Build history of the part. All positions in model axes, mm. Face numbers are marked on the shaded views. A direction names the side the tool comes from. Round coordinates to 2 decimals unless told otherwise and drop trailing zeros. Order: outer loops, then holes, each group sorted by start corner. A loop starts at its lowest first (then second) coordinate and runs counter-clockwise, first axis right, second up. Notation, with made-up numbers: (-11, 61.5) -> (-3, 61.5) arc R20 ccw to (-3, 88.5) -> close; hole circle Ø7 at (-16.75, -19). An arc over 180 degrees is marked (long way). Answer as a JSON object with one key per item and string values.
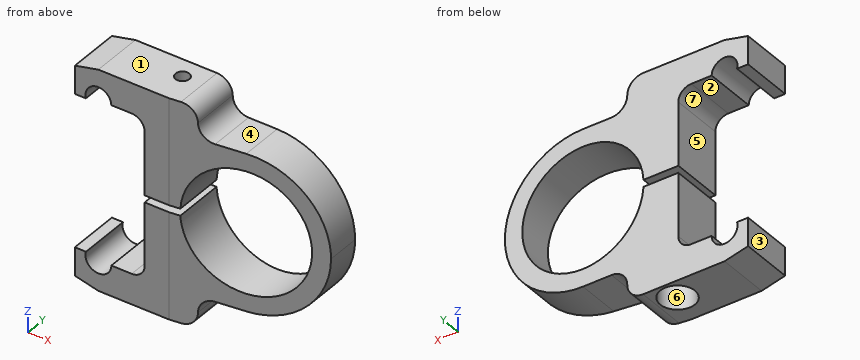
from build123d import *

# Parameters (mm, degrees)
F1_DEPTH       = 9.525
F3_D           = 2.54
F3_CBORE_D     = 6.35
F3_CBORE_DEPTH = 4.7752
F5_DEPTH       = 20.32


with BuildPart() as f1:
    # F0 (on Front) → F1 (new body)
    with BuildSketch(Plane.XZ):
        with BuildLine():
            ThreePointArc((-28.2059340648, 13.9065), (-26.240179578, 16.8438540599), (-23.5585, 14.5415))
            Line((-23.5585, 14.5415), (-19.8247, 14.5415))
            ThreePointArc((-19.8247, 14.5415), (-18.1543723615, 13.8496276385), (-17.4625, 12.1793))
            Line((-17.4625, 12.1793), (-17.4625, 0.6350352715))
            Line((-17.4625, 0.6350352715), (-11.0877819096, 0.6350352715))
            ThreePointArc((-11.0877819096, 0.6350352715), (11.0996948974, 3.52715e-05), (-11.0877819096, -0.6349647285))
            Line((-11.0877819096, -0.6349647285), (-17.4559396015, -0.6349647285))
            Line((-17.4559396015, -0.6349647285), (-17.4559396015, -12.1792647285))
            ThreePointArc((-17.4559396015, -12.1792647285), (-18.147811963, -13.8495923671), (-19.8181396015, -14.5414647285))
            Line((-19.8181396015, -14.5414647285), (-23.5519396015, -14.5414647285))
            ThreePointArc((-23.5519396015, -14.5414647285), (-26.2413382061, -16.9011545192), (-28.1991546105, -13.9065))
            Line((-28.1991546105, -13.9065), (-30.2311546105, -13.9065))
            Line((-30.2311546105, -13.9065), (-30.2311546105, -19.0742111302))
            Line((-30.2311546105, -19.0742111302), (-25.92066586, -20.0914))
            Line((-25.92066586, -20.0914), (-11.0116051104, -20.0914))
            ThreePointArc((-11.0116051104, -20.0914), (-8.9619217104, -19.2410649878), (-8.116123004, -17.1895055269))
            ThreePointArc((-8.116123004, -17.1895055269), (-7.2702919293, -15.137867554), (-5.220530089, -14.2875))
            Line((-5.220530089, -14.2875), (0, -14.2875))
            ThreePointArc((0, -14.2875), (10.1027881362, -10.1027881362), (14.2875, 0))
            ThreePointArc((14.2875, 0), (10.1027881362, 10.1027881362), (0, 14.2875))
            Line((0, 14.2875), (-5.220530089, 14.2875))
            ThreePointArc((-5.220530089, 14.2875), (-7.2612916673, 15.1288868805), (-8.1160675997, 17.1640767507))
            ThreePointArc((-8.1160675997, 17.1640767507), (-8.9646092373, 19.1930542961), (-10.9940030066, 20.0406))
            Line((-10.9940030066, 20.0406), (-25.92066586, 20.0406))
            Line((-25.92066586, 20.0406), (-30.2311546105, 19.0322602705))
            Line((-30.2311546105, 19.0322602705), (-30.2311546105, 13.9065))
            Line((-30.2311546105, 13.9065), (-28.2059340648, 13.9065))
        make_face()
    extrude(amount=F1_DEPTH)

    # F3 (through all)
    with Locations(Plane(origin=(0, 0, -20.0914), x_dir=(1, 0, 0), z_dir=(0, 0, -1))):
        with Locations((-14.6946051104, 3.683)):
            CounterBoreHole(F3_D / 2, F3_CBORE_D / 2, F3_CBORE_DEPTH)

    # F4 (on Top) → F5 (cut, symmetric)
    with BuildSketch(Plane.XY):
        Polygon((14.5003534853, -6.1715153816), (-13.6252772063, -9.5990113914), (14.5003534853, -10.0196320564), align=None)
    extrude(amount=F5_DEPTH, both=True, mode=Mode.SUBTRACT)


solid = f1.part
1) Cut at D-D, the plane z = -10.5. Give the cut face in (x, y) (3 decimals), plus the area to 3 significant figures.
Checked values:
{"outline": "(-17.456, -9.525) -> (-13.018, -9.525) -> (-3.612, -8.379) -> (-3.612, 0) -> (-17.456, 0) -> close; (3.605, -7.499) -> (9.689, -6.758) -> (9.689, 0) -> (3.605, 0) -> close; hole circle Ø2.54 at (-14.695, -3.683)", "area": "165 mm²"}
2) Probe L1, parallel to X at y = -3.25, z = -1.5; L2, parallel to X at y = -3.75, z = 6.5; L3, parallel to Z at x = -21.5, y = -3. List the from-to ranges inside material, lowest first. Write a range as from..to.
Checked values:
{"L1": "x = -17.46..-15.89, -13.5..-11, 11..14.21", "L2": "x = -17.46..-15.96, -13.43..-9, 9..12.72", "L3": "z = -20.09..-14.54, 14.54..20.04"}
3) Cut at C-C, the plane z = 13. Give the cut face in (x, y) (3 decimals), plus the area to 3 significant figures.
Checked values:
{"outline": "(-17.61, -9.525) -> (-13.018, -9.525) -> (5.927, -7.216) -> (5.927, 0) -> (-17.61, 0) -> close; hole circle Ø2.54 at (-14.695, -3.683)", "area": "197 mm²"}
4) Flat gauge pins, fed straight in: pin 1 Ø2 at (y, z) = (-1, 6.5) entering from +X; pin 2 Ø13.5 at (x, z) = (0, 0) entering from +Y; pin 3 Ø4 at (x, y) = (6, -8.5) entering from +Z; pin 4 Ø2 at (x, y) = (-29, -4.5) entering from -Z. Where does each tip first touch, or does it go through?
Checked values:
{"pin 1": "stops at x = 13.19", "pin 2": "passes through", "pin 3": "stops at z = 13.62", "pin 4": "stops at z = -19.6"}
5) Which spindle directions (+Z, -Z, +X, -X, +Y, -Y) get a long thin tool onto all of the face, cutting with end or side? Do the marked faces 4, 5, 6 and 7. Say none if no direction does.
Checked values:
{"face 4": "+Z, +X, +Y, -Y", "face 5": "-X, +Y, -Y", "face 6": "-Z", "face 7": "+Y, -Y"}
6) Pull direction Z, two halves, no side cores. Call the marked faces 1, 2 and 3: pulls with the +Z half, pulls with the -Z half, needs draft (parallel to the pull), parting line crosses it, or undercut.
Checked values:
{"face 1": "pulls with the +Z half", "face 2": "undercut", "face 3": "needs draft"}
7) Cut at B-B, the plane x = 4.5. Give the cut face in (y, z), plus the area to 3 significant figures.
Checked values:
{"outline": "(-7.39, -13.56) -> (0, -13.56) -> (0, -10.15) -> (-7.39, -10.15) -> close; (-7.39, 10.15) -> (0, 10.15) -> (0, 13.56) -> (-7.39, 13.56) -> close", "area": "50.4 mm²"}
8) Cut at A-A, the plane z = 3.5. Give the cut face in (x, y) (1 decimal).
Checked values:
{"outline": "(-17.5, -9.5) -> (-13, -9.5) -> (-10.5, -9.2) -> (-10.5, 0) -> (-17.5, 0) -> close; (10.5, -6.7) -> (13.9, -6.3) -> (13.9, 0) -> (10.5, 0) -> close; hole circle Ø2.5 at (-14.7, -3.7)"}
